Autodesk Inventor part; units mm, degrees
ref_plane "YZ Plane" through (0, 0, 0) normal (1, 0, 0) x (0, 1, 0)
ref_plane "XZ Plane" through (0, 0, 0) normal (0, 1, 0) x (-1, 0, 0)
ref_plane "XY Plane" through (0, 0, 0) normal (0, 0, 1) x (1, 0, 0)
sketch "Sketch1" plane through (0, 0, 0) normal (0, 1, 0) x (-1, 0, 0)
  line L0 (2, 2) -> (-2, 2)
  line L1 (-2, 2) -> (-2, -2)
  line L2 (-2, -2) -> (2, -2)
  line L3 (2, -2) -> (2, 2)
  line L4 (2, 2) -> (-2, -2) construction
  line L5 (-2, 2) -> (2, -2) construction
  circle A0 centre (0, 0) radius 0.75
  dimension "d0" = 4
  dimension "d1" = 4
  dimension "d2" = 1.5
extrude "Extrusion1" add sketch "Sketch1" along normal blind 10
sketch "Sketch2" plane through (0, 10, 0) normal (0, 1, 0) x (1, 0, 0)
  line L0 (-1.5, 1.5) -> (1.5, -1.5) construction
  line L1 (1.5, 1.5) -> (-1.5, -1.5) construction
  circle A0 centre (1.5, -1.5) radius 0.225
  circle A1 centre (1.5, 1.5) radius 0.225
  circle A2 centre (-1.5, 1.5) radius 0.225
  circle A3 centre (-1.5, -1.5) radius 0.225
  point P0 (0, 0)
  dimension "d5" = 3
  dimension "d7" = 0.45
  dimension "d8" = 0.45
  dimension "d9" = 0.45
  dimension "d10" = 0.45
extrude "Extrusion2" add sketch "Sketch2" along normal blind 1
sketch "Sketch3" plane through (0, 0, 0) normal (0, -1, 0) x (1, 0, 0)
  line L0 (1, 0.25) -> (-1, 0.25)
  line L1 (-1, 0.25) -> (-1, -0.25)
  line L2 (-1, -0.25) -> (1, -0.25)
  line L3 (1, -0.25) -> (1, 0.25)
  line L4 (1, 0.25) -> (-1, -0.25) construction
  line L5 (-1, 0.25) -> (1, -0.25) construction
  point P0 (0, 0)
  dimension "d13" = 2
  dimension "d14" = 0.5
extrude "Extrusion3" add sketch "Sketch3" against normal blind 0.5
fillet "Fillet1" radius 0.25 4 edges at (0, 0, 0.25) (0, 0, -0.25) (0, 0.5, 0.25) (0, 0.5, -0.25)
properties part number "SpringAttachment"
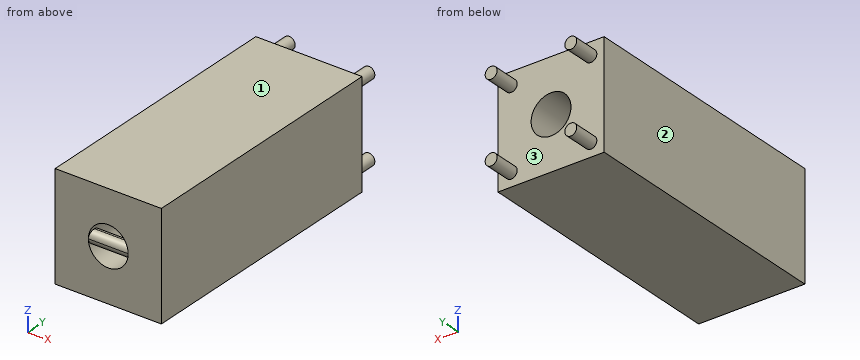
For this review, take the finished solid that the model builds, in its own axes (mm). Face numbers are marked on the shaded views. Give positions to 0.01 mm unless a question says otherwise; leave off trailing zeros. Order: outer loops, then holes, each group sorted by start corner. A loop starts at its lowest first (then second) coordinate and runs counter-clockwise, first axis right, second up. Notation, with made-up numbers: (81, 8) - (120, 8) arc R19 cw to (120, 34) - close; hole circle Ø7 at (-0.5, 25.25). An arc over 180 degrees is marked (long way). Answer as a JSON object with one key per item and string values. Group by question number.
Item 1: Take a section at B-B on y = 5.5. Give the boundary of the cut face in (x, z), and give its area (3 significant figures).
Item 2: Clearance check with flat-ended pins moving along their axes: pin 1 Ø1.2 at (x, z) = (-0.5, 1) entering from +Y; pin 2 Ø1.4 at (x, z) = (0, 0) entering from +Y; pin 3 Ø1 at (x, z) = (-1.5, -1.5) entering from -Y. State where each tip first meets the part, or that it passes through.
Item 3: Take a section at D-D on z = 0.4. Give the boundary of the cut face in (x, y).
Item 4: Draft analysis for pull direction Z (two halves, no side actions). For the marked faces 1, 2 and 3, state which applies: pulls with the +Z half, pulls with the -Z half, needs draft (parallel to the pull), parting line crosses it, or undercut.
Item 5: Take a section at A-A on x = 0. Give the number of separate pieces and of enclosed holes in the cut face, and give its area (3 significant figures).
Item 6: Take a section at C-C on x = -1.5. Give the boundary of the cut face in (y, z) (3 decimals).
Item 7: Wall thickness on line 1 along Z through (x, y) = (0, 8); line 2 along Y through (x, z) = (0.25, 1.1): over which ranges is each line inside the solid? List them lowest first.
Reported:
{
 "1": {"outline": "(-2, -2) - (2, -2) - (2, 2) - (-2, 2) - close; hole circle Ø1.5 at (0, 0)", "area": "14.2 mm^2"},
 "2": {"pin 1": "y = 10", "pin 2": "y = 0.5", "pin 3": "y = 0"},
 "3": {"outline": "(-2, 0) - (-0.63, 0) - (-0.63, 10) - (-2, 10) - close; (0.63, 0) - (2, 0) - (2, 10) - (0.63, 10) - close"},
 "4": {"face 1": "pulls with the +Z half", "face 2": "needs draft", "face 3": "undercut"},
 "5": {"separate pieces": "3", "enclosed holes": "0", "area": "25.2 mm^2"},
 "6": {"outline": "(0, -2) - (10, -2) - (10, -1.725) - (11, -1.725) - (11, -1.275) - (10, -1.275) - (10, 1.275) - (11, 1.275) - (11, 1.725) - (10, 1.725) - (10, 2) - (0, 2) - close"},
 "7": {"line 1": "-2 to -0.75, 0.75 to 2", "line 2": "0 to 10"}
}
